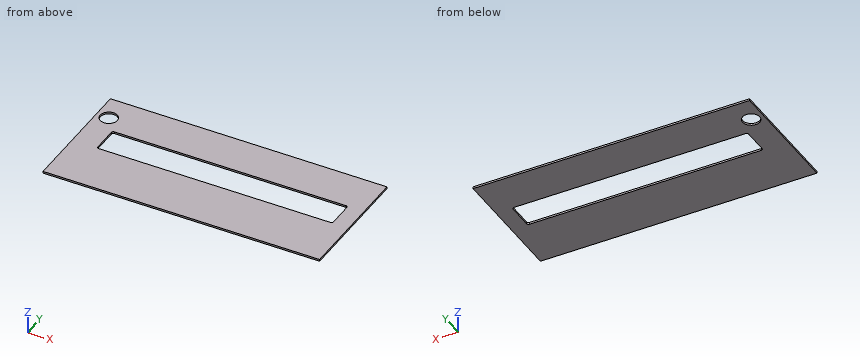
```python
from build123d import *

# Parameters (mm, degrees)
F0_W     = 145
F0_H     = 65
F0_R     = 4.5
F1_DEPTH = 1


with BuildPart() as f1:
    # F0 (on Top) → F1 (new body)
    with BuildSketch(Plane.XY):
        with Locations((72.5, 32.5)):
            Rectangle(F0_W, F0_H)
        with Locations((6.5, 51.5)):
            Circle(F0_R, mode=Mode.SUBTRACT)
        with BuildLine():
            ThreePointArc((13, 42), (13.292893, 42.707107), (14, 43))
            Line((14, 43), (135.5, 43))
            ThreePointArc((135.5, 43), (136.207107, 42.707107), (136.5, 42))
            Line((136.5, 42), (136.5, 29))
            ThreePointArc((136.5, 29), (136.207107, 28.292893), (135.5, 28))
            Line((135.5, 28), (14, 28))
            ThreePointArc((14, 28), (13.292893, 28.292893), (13, 29))
            Line((13, 29), (13, 42))
        make_face(mode=Mode.SUBTRACT)
    extrude(amount=F1_DEPTH)


solid = f1.part
```
Verification items for the finished model (mm, model axes). Give positions to 0.01 mm unless a question says otherwise; leave off trailing zeros. Order: outer loops, then holes, each group sorted by start corner. A loop starts at its lowest first (then second) coordinate and runs counter-clockwise, first axis right, second up. Notation, with made-up numbers: M 82.5,-18 L 130.5,-18 A18 ccw 130.5,8 Z; hole C 41,79.25 d6. An arc over 180 degrees is marked long. Return JSON: item names as keys, results as strings. Group by question number.
1) Scan lines: line 1 (Y direction, x = 49.5, z = 0.6); line 2 (Y direction, x = 6.5, z = 0.35); line 3 (X direction, y = 40, z = 0.45). Record each from-to range of solid material in increasing order.
2) Section check B-B on z = 0.4. Record the cut outline in (x, y), and give its area (3 significant figures).
3) Section check C-C on x = 63. Record the cut outline in (y, z).
4) Section check A-A on x = 6.5. Record the cut outline in (y, z).
5) Go/stop test with flat-tipped pins: pin 1 Ø4 at (x, y) = (39.5, 52.5) entering from -Z; pin 2 Ø8 at (x, y) = (6.5, 51.5) entering from -Z. Record where each tip stops, or that it passes through.
Answer block:
{
 "1": {"line 1": "y = 0 to 28, 43 to 65", "line 2": "y = 0 to 47, 56 to 65", "line 3": "x = 0 to 13, 136.5 to 145"},
 "2": {"outline": "M 0,0 L 145,0 L 145,65 L 0,65 Z; hole C 6.5,51.5 d9; hole M 13,29 A1 ccw 14,28 L 135.5,28 A1 ccw 136.5,29 L 136.5,42 A1 ccw 135.5,43 L 14,43 A1 ccw 13,42 Z", "area": "7,510 mm^2"},
 "3": {"outline": "M 0,0 L 28,0 L 28,1 L 0,1 Z; M 43,0 L 65,0 L 65,1 L 43,1 Z"},
 "4": {"outline": "M 0,0 L 47,0 L 47,1 L 0,1 Z; M 56,0 L 65,0 L 65,1 L 56,1 Z"},
 "5": {"pin 1": "stops at z = 0", "pin 2": "passes through"}
}
